Here's how the part is built. I have some questions about the finished solid (model axes, mm). Face numbers are marked on the shaded views. A direction names the side the tool comes from. Give positions to 0.01 mm unless a question says otherwise; leave off trailing zeros. Loops run counter-clockwise (first coordinate to the right, second up) from the corner with the lowest first, then second, coordinate; pieces in that order, holes last. Notation, with made-up numbers: (0, 86.25) - (35, 86.25) arc R11 ccw to (35, 93.25) - close; hole circle Ø11 at (-11.5, -29.75). An arc over 180 degrees is marked (long way). Use one line per item in the form item = value.
from build123d import *

# Parameters (mm, degrees)
BOSS_EXTRUDE1_DEPTH                               = 12.7
CUT_EXTRUDE1_DEPTH                                = 45.522766139
CUT_EXTRUDE1_DEPTH_BACK                           = 45.522766139
SKETCH2_R                                         = 83.82
BOSS_EXTRUDE2_DEPTH                               = 7.9375
CHAMFER1_SIZE                                     = 6.35
CSK_FOR_8_FLAT_HEAD_MACHINE_SCREW_100_D           = 4.4958
CSK_FOR_8_FLAT_HEAD_MACHINE_SCREW_100_CSINK_D     = 8.4328
CSK_FOR_8_FLAT_HEAD_MACHINE_SCREW_100_CSINK_ANGLE = 100
SKETCH6_R                                         = 1.631947848
SKETCH6_R_2                                       = 1.523937663
CUT_EXTRUDE2_DEPTH                                = 38.304291688
SKETCH7_W                                         = 1.5875
SKETCH7_H                                         = 1.190625
CUT_EXTRUDE3_DEPTH                                = 35.276937503
SKETCH8_R                                         = 4.7625
SKETCH8_R_2                                       = 3.81
CUT_EXTRUDE4_DEPTH                                = 38.304291688
CHAMFER2_SIZE                                     = 0.508


with BuildPart() as part:
    # Sketch1 → Boss-Extrude1 (new body)
    with BuildSketch(Plane(origin=(0, 0, 0), x_dir=(1, 0, 0), z_dir=(0, 1, 0))):
        Polygon((-28.511825699, 12.845271113), (-22.161825699, 19.195271113), (-9.461825699, 19.195271113), (-3.111825699, 12.845271113), (-3.111825699, -12.554728887), (-28.511825699, -12.554728887), align=None)
    extrude(amount=BOSS_EXTRUDE1_DEPTH)

    # Sketch2 → Cut-Extrude1 (cut, two sides: drawn at the far end of the back side and taken through both)
    with BuildSketch(Plane.XY.offset(12.554728887).offset(-CUT_EXTRUDE1_DEPTH_BACK)):
        with Locations((-15.811825699, -82.852292666)):
            Circle(SKETCH2_R)
    extrude(amount=CUT_EXTRUDE1_DEPTH + CUT_EXTRUDE1_DEPTH_BACK, mode=Mode.SUBTRACT)

    # Sketch5 → Boss-Extrude2 (add)
    with BuildSketch(Plane(origin=(0, 0, -19.195271113), x_dir=(-1, 0, 0), z_dir=(0, 0, -1))):
        with BuildLine():
            Line((3.111825699, 12.7), (3.111825699, 0))
            Line((3.111825699, 0), (3.111825699, -1.799225087))
            ThreePointArc((3.111825699, -1.799225087), (15.811825699, -0.810292666), (28.511825699, -1.799225087))
            Line((28.511825699, -1.799225087), (28.511825699, 0))
            Line((28.511825699, 0), (28.511825699, 12.7))
            Line((28.511825699, 12.7), (3.111825699, 12.7))
        make_face()
    extrude(amount=-BOSS_EXTRUDE2_DEPTH)

    # Chamfer1
    chamfer1_edges = [part.edges().sort_by_distance(p)[0] for p in [
        (-3.111825699, 5.450387457, -19.195271113),
        (-28.511825699, 5.450387457, -19.195271113),
    ]]
    chamfer(chamfer1_edges, length=CHAMFER1_SIZE)

    # CSK for #8 Flat Head Machine Screw (100)1 (through all)
    with Locations(Plane(origin=(0, 12.7, 0), x_dir=(1, 0, 0), z_dir=(0, 1, 0))):
        with Locations((-20.177450699, 14.432771113), (-11.446200699, 14.432771113)):
            CounterSinkHole(CSK_FOR_8_FLAT_HEAD_MACHINE_SCREW_100_D / 2, CSK_FOR_8_FLAT_HEAD_MACHINE_SCREW_100_CSINK_D / 2, counter_sink_angle=CSK_FOR_8_FLAT_HEAD_MACHINE_SCREW_100_CSINK_ANGLE)

    # Sketch6 → Cut-Extrude2 (cut, through all)
    with BuildSketch(Plane(origin=(0, 12.7, 0), x_dir=(1, 0, 0), z_dir=(0, 1, 0))):
        with Locations(Location((-15.811825699, 7.130260145, 0), (0, 0, 270))):
            Circle(SKETCH6_R)
        with Locations(Location((-15.811825699, -2.775791253, 0), (0, 0, 270))):
            Circle(SKETCH6_R_2)
    extrude(amount=-CUT_EXTRUDE2_DEPTH, mode=Mode.SUBTRACT)

    # Sketch7 → Cut-Extrude3 (cut, through all)
    with BuildSketch(Plane.ZY.offset(28.511825699)):
        with Locations((-10.464021113, 0.5953125)):
            Rectangle(SKETCH7_W, SKETCH7_H)
    extrude(amount=-CUT_EXTRUDE3_DEPTH, mode=Mode.SUBTRACT)

    # Sketch8 → Cut-Extrude4 (cut, through all)
    with BuildSketch(Plane(origin=(0, 12.7, 0), x_dir=(1, 0, 0), z_dir=(0, 1, 0))):
        with Locations(Location((-15.811825699, -2.775791253, 0), (0, 0, 270))):
            Circle(SKETCH8_R)
        with Locations(Location((-15.811825699, 7.130260145, 0), (0, 0, 270))):
            Circle(SKETCH8_R_2)
    extrude(amount=-CUT_EXTRUDE4_DEPTH, mode=Mode.SUBTRACT)

    # Chamfer2
    # the kernel refuses this chamfer: 0.508 mm, written as the material it takes off along each edge
    with BuildSketch(Plane(origin=(-15.811825699, 12.7, 2.775791253), x_dir=(0, 0, 1), z_dir=(-1, 0, 0))) as chamfer2_piece_1:
        Polygon((4.7625 + CHAMFER2_SIZE, 0), (4.7625, -CHAMFER2_SIZE), (4.7625, 0), align=None)
    revolve(axis=Axis((-15.811825699, 12.7, 2.775791253), (0, 1, 0)), mode=Mode.SUBTRACT)
    with BuildSketch(Plane(origin=(-15.811825699, 12.7, -7.130260145), x_dir=(0, 0, 1), z_dir=(-1, 0, 0))) as chamfer2_piece_2:
        Polygon((3.81 + CHAMFER2_SIZE, 0), (3.81, -CHAMFER2_SIZE), (3.81, 0), align=None)
    revolve(axis=Axis((-15.811825699, 12.7, -7.130260145), (0, 1, 0)), mode=Mode.SUBTRACT)


solid = part.part
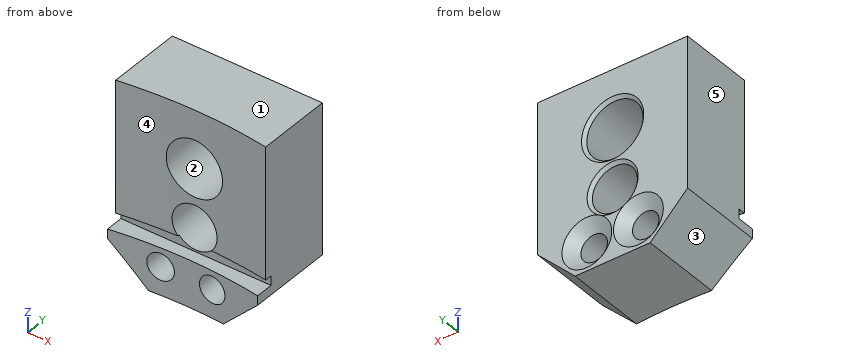
(1) If we section it at B-B (x = -26.5): List the corners of the cut face in (y, z) for me.
Geometry says:
outline = (-1.51, -14.86) - (12.7, -14.86) - (12.7, 12.55) - (0.28, 12.55) - (0.28, -9.67) - (1.19, -9.67) - (1.19, -11.26) - (-1.51, -11.26) - close
(2) For P1, Ø1.5, axis at y = 3.5, z = -16, coming from the +X side; P2, Ø0.5, axis at x = -10, z = -10, coming from the -Y side; P3, Ø12, axis at x = -13.5, z = 4.5, coming from the -Y side, each with a flat end and sliding along its axis, tell me the tip position at first contact or that it passes through.
Geometry says:
P1 = -5.52
P2 = 1.19
P3 = 0.55
(3) If we section it at C-C (x = -17.25): Give the number of separate pieces and of enclosed holes in the cut face, plus the area to 3 significant figures.
Geometry says:
separate_pieces = 3
enclosed_holes = 0
area = 193 mm²
(4) Thinking about a two-plate mould opening in X: for the marked faces 1, 2 and 3, which applies, pulls with the +X half, pulls with the -X half, needs draft (parallel to the pull), parting line crosses it, or undercut?
Geometry says:
face_1 = needs draft
face_2 = undercut
face_3 = pulls with the -X half
(5) For the marked faces 4 and 5, which set-ups out of +Z, -Z, +X, -X, +Y, -Y let a thin tool reach every point of the face, with its end or its side?
Geometry says:
face_4 = +Z, -Y
face_5 = +Z, -Z, -X, +Y, -Y
(6) If I drill on probe 1 along Z at (x, y) = (-15.75, 1); probe 2 along Z at (x, y) = (-13.25, 10.25); probe 3 along X at (y, z) = (4.75, -16.5), over which ranges is the centre line in solid material (lowest first)?
Geometry says:
probe_1 = -19.2 to -11.26, -3.32 to -1.99, 7.54 to 12.55
probe_2 = -19.2 to -15.77, -13.09 to -9.95, -4.31 to -1.24, 6.79 to 12.55
probe_3 = -24.86 to -21.06, -19.29 to -12.33, -10.56 to -6.77
(7) If we section it at A-A (y = 1.75): List the corners of the cut face in (x, z) for me (1 decimal).
Geometry says:
outline = (-28.5, -12.8) - (-22.2, -19.2) - (-9.5, -19.2) - (-3.1, -12.8) - (-3.1, 12.6) - (-28.5, 12.6) - close; hole circle Ø4.5 at (-20.2, -14.4); hole circle Ø9.5 at (-15.8, 2.8); hole circle Ø7.6 at (-15.8, -7.1); hole circle Ø4.5 at (-11.4, -14.4)
